```python
from build123d import *

# Parameters (mm, degrees)
SKETCH_1_W      = 180
SKETCH_1_H      = 90
SKETCH_1_W_2    = 10
SKETCH_1_H_2    = 3
SKETCH_1_W_3    = 3
SKETCH_1_H_3    = 10
EXTRUDE_1_DEPTH = 3


with BuildPart() as part:
    # 草图1 → 凸台-拉伸1 (new body)
    with BuildSketch(Plane.XY):
        with Locations((-0.098158541, -0.288232222)):
            Rectangle(SKETCH_1_W, SKETCH_1_H)
        with Locations((-75.098158541, 41.211767778)):
            Rectangle(SKETCH_1_W_2, SKETCH_1_H_2, mode=Mode.SUBTRACT)
        with Locations((-86.598158541, 29.711767778)):
            Rectangle(SKETCH_1_W_3, SKETCH_1_H_3, mode=Mode.SUBTRACT)
        with Locations((-86.598158541, 14.711767778)):
            Rectangle(SKETCH_1_W_3, SKETCH_1_H_3, mode=Mode.SUBTRACT)
        with Locations((-86.598158541, -0.288232222)):
            Rectangle(SKETCH_1_W_3, SKETCH_1_H_3, mode=Mode.SUBTRACT)
        with Locations((-86.598158541, -15.288232222)):
            Rectangle(SKETCH_1_W_3, SKETCH_1_H_3, mode=Mode.SUBTRACT)
        with Locations((-86.598158541, -30.288232222)):
            Rectangle(SKETCH_1_W_3, SKETCH_1_H_3, mode=Mode.SUBTRACT)
        with Locations((86.401841459, -30.288232222)):
            Rectangle(SKETCH_1_W_3, SKETCH_1_H_3, mode=Mode.SUBTRACT)
        with Locations((86.401841459, -15.288232222)):
            Rectangle(SKETCH_1_W_3, SKETCH_1_H_3, mode=Mode.SUBTRACT)
        with Locations((86.401841459, -0.288232222)):
            Rectangle(SKETCH_1_W_3, SKETCH_1_H_3, mode=Mode.SUBTRACT)
        with Locations((86.401841459, 14.711767778)):
            Rectangle(SKETCH_1_W_3, SKETCH_1_H_3, mode=Mode.SUBTRACT)
        with Locations((86.401841459, 29.711767778)):
            Rectangle(SKETCH_1_W_3, SKETCH_1_H_3, mode=Mode.SUBTRACT)
        with Locations((-60.098158541, 41.211767778)):
            Rectangle(SKETCH_1_W_2, SKETCH_1_H_2, mode=Mode.SUBTRACT)
        with Locations((-45.098158541, 41.211767778)):
            Rectangle(SKETCH_1_W_2, SKETCH_1_H_2, mode=Mode.SUBTRACT)
        with Locations((-30.098158541, 41.211767778)):
            Rectangle(SKETCH_1_W_2, SKETCH_1_H_2, mode=Mode.SUBTRACT)
        with Locations((-15.098158541, 41.211767778)):
            Rectangle(SKETCH_1_W_2, SKETCH_1_H_2, mode=Mode.SUBTRACT)
        with Locations((-0.098158541, 41.211767778)):
            Rectangle(SKETCH_1_W_2, SKETCH_1_H_2, mode=Mode.SUBTRACT)
        with Locations((14.901841459, 41.211767778)):
            Rectangle(SKETCH_1_W_2, SKETCH_1_H_2, mode=Mode.SUBTRACT)
        with Locations((29.901841459, 41.211767778)):
            Rectangle(SKETCH_1_W_2, SKETCH_1_H_2, mode=Mode.SUBTRACT)
        with Locations((44.901841459, 41.211767778)):
            Rectangle(SKETCH_1_W_2, SKETCH_1_H_2, mode=Mode.SUBTRACT)
        with Locations((59.901841459, 41.211767778)):
            Rectangle(SKETCH_1_W_2, SKETCH_1_H_2, mode=Mode.SUBTRACT)
        with Locations((74.901841459, 41.211767778)):
            Rectangle(SKETCH_1_W_2, SKETCH_1_H_2, mode=Mode.SUBTRACT)
        with Locations((74.901841459, -41.788232222)):
            Rectangle(SKETCH_1_W_2, SKETCH_1_H_2, mode=Mode.SUBTRACT)
        with Locations((59.901841459, -41.788232222)):
            Rectangle(SKETCH_1_W_2, SKETCH_1_H_2, mode=Mode.SUBTRACT)
        with Locations((44.901841459, -41.788232222)):
            Rectangle(SKETCH_1_W_2, SKETCH_1_H_2, mode=Mode.SUBTRACT)
        with Locations((29.901841459, -41.788232222)):
            Rectangle(SKETCH_1_W_2, SKETCH_1_H_2, mode=Mode.SUBTRACT)
        with Locations((14.901841459, -41.788232222)):
            Rectangle(SKETCH_1_W_2, SKETCH_1_H_2, mode=Mode.SUBTRACT)
        with Locations((-0.098158541, -41.788232222)):
            Rectangle(SKETCH_1_W_2, SKETCH_1_H_2, mode=Mode.SUBTRACT)
        with Locations((-15.098158541, -41.788232222)):
            Rectangle(SKETCH_1_W_2, SKETCH_1_H_2, mode=Mode.SUBTRACT)
        with Locations((-30.098158541, -41.788232222)):
            Rectangle(SKETCH_1_W_2, SKETCH_1_H_2, mode=Mode.SUBTRACT)
        with Locations((-45.098158541, -41.788232222)):
            Rectangle(SKETCH_1_W_2, SKETCH_1_H_2, mode=Mode.SUBTRACT)
        with Locations((-60.098158541, -41.788232222)):
            Rectangle(SKETCH_1_W_2, SKETCH_1_H_2, mode=Mode.SUBTRACT)
        with Locations((-75.098158541, -41.788232222)):
            Rectangle(SKETCH_1_W_2, SKETCH_1_H_2, mode=Mode.SUBTRACT)
    extrude(amount=EXTRUDE_1_DEPTH)


solid = part.part
```
Geometry: final body of the model. Coordinates: model frame, mm. Round coordinates to 2 decimals unless told otherwise and drop trailing zeros. Order: outer loops, then holes, each group sorted by start corner. A loop starts at its lowest first (then second) coordinate and runs counter-clockwise, first axis right, second up. Notation, with made-up numbers: M 50.25,22.5 L 108.25,22.5 A17 ccw 108.25,38.5 Z; hole C -7.75,-27 d4. An arc over 180 degrees is marked long. One line per item, written item: value.
(1) Cut plane C-C (z = 2.25). Give the number of separate pieces and of enclosed holes in the cut face, and give its area (3 significant figures).
Result sheet:
separate pieces: 1
enclosed holes: 32
area: 15,200 mm2
(2) Line query: probe 1 along Y at (x, z) = (-14, 1.55); probe 2 along X at (y, z) = (28.5, 2.45). Output: solid intervals per line, ascending. Write a range as [from, to].
Result sheet:
probe 1: [-45.29, -43.29], [-40.29, 39.71], [42.71, 44.71]
probe 2: [-90.1, -88.1], [-85.1, 84.9], [87.9, 89.9]
(3) Cut plane A-A (y = 0). Return the cut outline in (x, z).
Result sheet:
outline: M -90.1,0 L -88.1,0 L -88.1,3 L -90.1,3 Z; M -85.1,0 L 84.9,0 L 84.9,3 L -85.1,3 Z; M 87.9,0 L 89.9,0 L 89.9,3 L 87.9,3 Z
(4) Cut plane B-B (x = 33). Return the cut outline in (y, z), and give its area (3 significant figures).
Result sheet:
outline: M -45.29,0 L -43.29,0 L -43.29,3 L -45.29,3 Z; M -40.29,0 L 39.71,0 L 39.71,3 L -40.29,3 Z; M 42.71,0 L 44.71,0 L 44.71,3 L 42.71,3 Z
area: 252 mm2
